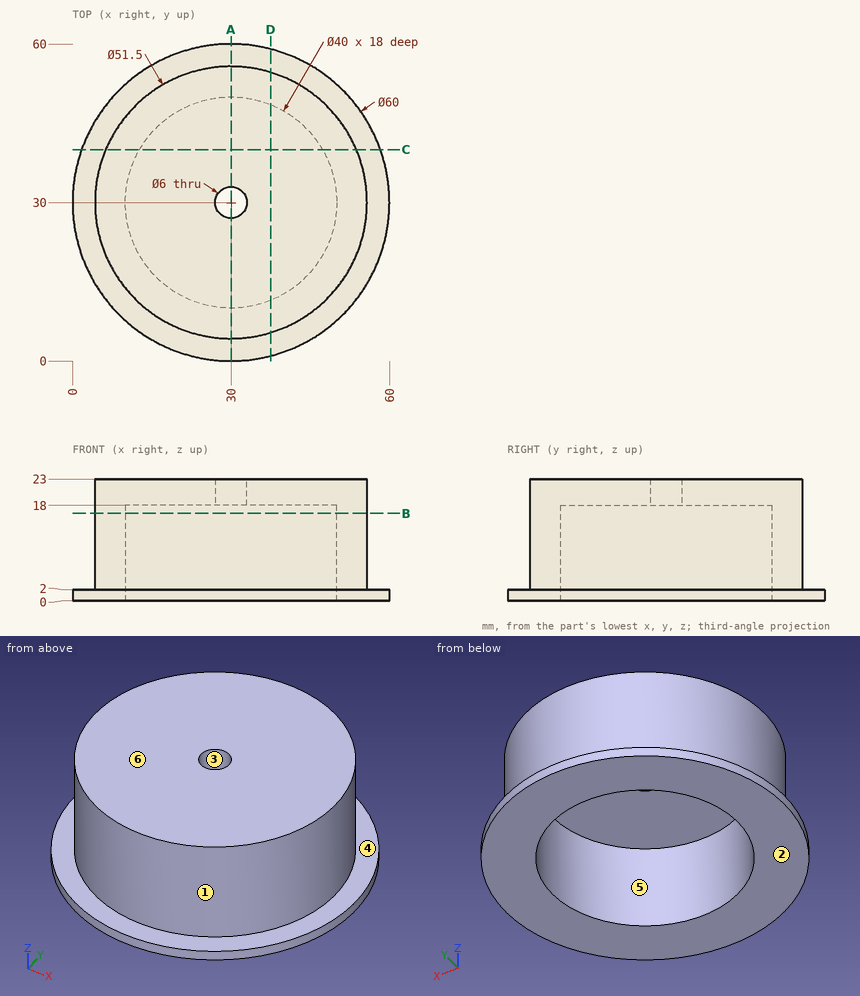
Can you work these out from the drawing? Everything is in mm from the part's minimum corner. A direction names the side the tool comes from. Give positions to 0.01 mm unless a question says otherwise; leave off trailing zeros. Loops run counter-clockwise (first coordinate to the right, second up) from the corner with the lowest first, then second, coordinate; pieces in that order, holes last. Notation, with made-up numbers: (-20.5, 9.25) -> (-12.5, 9.25) arc R26 cw to (-12.5, 37.25) -> close; hole circle Ø9 at (9, 77.25). An arc over 180 degrees is marked (long way). Put each result on its own line as item: value.
(1) Imagine slicing it at C-C on y = 40. Write out the boundary of the cut face in (x, z), plus the area to 3 significant figures.
Computed:
outline: (1.72, 0) -> (12.68, 0) -> (12.68, 18) -> (47.32, 18) -> (47.32, 0) -> (58.28, 0) -> (58.28, 2) -> (53.73, 2) -> (53.73, 23) -> (6.27, 23) -> (6.27, 2) -> (1.72, 2) -> close
area: 486 mm^2
(2) Please list where these lines run through material, in increasing order: probe 1 along Y at (x, z) = (30, 11.5); probe 2 along Z at (x, y) = (3, 19.5); probe 3 along Y at (x, z) = (23, 7.5) (3 decimals). Write a range as [from, to].
Computed:
probe 1: [4.25, 10], [50, 55.75]
probe 2: [0, 2]
probe 3: [5.22, 11.265], [48.735, 54.78]
(3) Thinking about a two-plate mould opening in X: for the marked faces 1, 2 and 3, which applies, pulls with the +X half, pulls with the -X half, needs draft (parallel to the pull), parting line crosses it, or undercut?
Computed:
face 1: parting line crosses it
face 2: needs draft
face 3: undercut
(4) Imagine slicing it at A-A on x = 30. Write out the boundary of the cut face in (y, z), plus the area to 4 significant figures.
Computed:
outline: (0, 0) -> (10, 0) -> (10, 18) -> (27, 18) -> (27, 23) -> (4.25, 23) -> (4.25, 2) -> (0, 2) -> close; (33, 18) -> (50, 18) -> (50, 0) -> (60, 0) -> (60, 2) -> (55.75, 2) -> (55.75, 23) -> (33, 23) -> close
area: 451.5 mm^2
(5) Imagine slicing it at B-B on z = 16.5. Write out the boundary of the cut face in (x, y), plus the area to 3 significant figures.
Computed:
outline: circle Ø51.5 at (30, 30); hole circle Ø40 at (30, 30)
area: 826 mm^2
(6) For the marked faces 4, 5 and 6, which set-ups out of +Z, -Z, +X, -X, +Y, -Y let a thin tool reach every point of the face, with its end or its side?
Computed:
face 4: +Z
face 5: -Z
face 6: +Z, +X, -X, +Y, -Y
(7) Imagine slicing it at D-D on x = 37.5. Write out the boundary of the cut face in (y, z), plus the area to 3 significant figures.
Computed:
outline: (0.95, 0) -> (11.46, 0) -> (11.46, 18) -> (48.54, 18) -> (48.54, 0) -> (59.05, 0) -> (59.05, 2) -> (54.63, 2) -> (54.63, 23) -> (5.37, 23) -> (5.37, 2) -> (0.95, 2) -> close
area: 483 mm^2
(8) I'm going to push flat-ended pins straight in: pin 1 Ø12 at (x, y) = (31.5, 26) entering from -Z; pin 2 Ø5 at (x, z) = (50, 10.5) entering from +Y; pin 3 Ø10 at (y, z) = (39, 9.5) entering from +X. Where does each tip first touch, or does it pass through?
Computed:
pin 1: z = 18
pin 2: y = 48.89
pin 3: x = 55.44
